The listing builds one solid part. Answer for the finished solid, in the listing's coordinates (mm). A direction names the side the tool comes from. Give positions to 0.01 mm unless a question says otherwise; leave off trailing zeros. Write each loop counter-clockwise with the first axis right and the second up, starting at its lowest first coordinate (ties: lowest second). Pieces come first, ordered by that corner, then holes. Notation, with made-up numbers: (-23, 19.25) - (10, 19.25) arc R34 ccw to (10, 50.25) - close; hole circle Ø4 at (81, 68.25). An arc over 180 degrees is marked (long way). Return JSON: item names as keys, results as strings.
Autodesk Inventor part; units mm, degrees
ref_plane "YZ Plane" through (0, 0, 0) normal (1, 0, 0) x (0, 1, 0)
ref_plane "XZ Plane" through (0, 0, 0) normal (0, 1, 0) x (-1, 0, 0)
ref_plane "XY Plane" through (0, 0, 0) normal (0, 0, 1) x (1, 0, 0)
sketch "スケッチ1" plane through (0, 0, 0) normal (0, 0, 1) x (1, 0, 0)
  circle A0 centre (0, 0) radius 17
  circle A1 centre (0, 0) radius 12
  circle A2 centre (0, -160) radius 12
  line L0 (-12, 0) -> (10.75, 0)
  line L1 (12, -160) -> (11, -160)
  circle A3 centre (0, -160) radius 17
  line L2 (-10, 24.6876) -> (10, 24.6876)
  line L3 (10, 24.6876) -> (10, -208.9864)
  line L4 (10, -208.9864) -> (-10, -208.9864)
  line L5 (-10, -208.9864) -> (-10, 24.6876)
  point P0 (-8, 8.9443)
  point P1 (12, 0)
  point P2 (0, -167.6676)
  point P3 (9.375, -145.8187)
  point P4 (-10.625, -146.7294)
  point P5 (-10.625, -13.2706)
  point P6 (9.375, -14.1813)
  point P7 (-0.625, 0)
  point P8 (-10, -13.7477)
  point P9 (-10, -146.2523)
  point P10 (10, -146.2523)
  point P11 (10, -13.7477)
  point P12 (10, -173.7477)
  point P13 (-10, -173.7477)
  point P14 (-10, 13.7477)
  point P15 (10, 13.7477)
  point P16 (-10, 6.6332)
  point P17 (-10, 0)
  point P18 (10, 0)
  point P19 (10, 6.6332)
  point P20 (-10, -6.6332)
  point P21 (10, -6.6332)
  point P22 (-10, -153.3668)
  point P23 (-10, -166.6332)
  point P24 (10, -166.6332)
  point P25 (10, -153.3668)
  dimension "d17" = 24
  dimension "d0" = 34
  dimension "d1" = 24
  dimension "d22" = 160
  dimension "d24" = 0
  dimension "d27" = 34
  dimension "d31" = 10
  dimension "d32" = 20
extrude "押し出し1" add sketch "スケッチ1" along normal blind 8 contours A0 L3 A1 | L3 A1 L5 A0 | L3 A3 L5 A0 | A0 L5 A1 L3 | L5 A1 A0 | L3 A2 L5 A3 | A3 L3 A2 | L5 A2 A3 | L5 A2 L3 A3
fillet "フィレット2" radius 5 4 edges at (-10, -146.2523, 4) (10, -146.2523, 4) (10, -13.7477, 4) (-10, -13.7477, 4)
equation "\"d17\" = d1"
equation "\"d31\" = 0.5 * d32"
equation "\"d23\" = 0.5 * d3"
properties part number "RP_Thigh-Link" material "アルミニウム7075"
Item 1: For faces 3 (the face through (10, -79, 4)), 4 (the face through (0.57, -176.99, 3.94)), 5 (the face through (-10.4, -14.13, 4.06)), determine the directions among +Z, -Z, +X, -X, +Y, -Y from which every point of the face is accessible in a straight line to the end or side of a thin tool.
Answer below:
{"face 3": "+Z, -Z, +X", "face 4": "+Z, -Z", "face 5": "+Z, -Z, -X"}
Item 2: The mould has two halves that part along Y. Classify faces 1 (the face through (0, -79, 0)), 2 (the face through (-10.426, -145.927, 4.056)): +Y half, -Y half, draft (parallel to the pull), parting line (faces both ways), or undercut.
Answer below:
{"face 1": "draft", "face 2": "undercut"}
Item 3: A cutting plane is placed at D-D on y = -102.5. Determine the outline of the cut face in (x, z), then the cut area to 3 significant figures.
Answer below:
{"outline": "(-10, 0) - (10, 0) - (10, 8) - (-10, 8) - close", "area": "160 mm²"}
Item 4: A cutting plane is placed at B-B on x = 0. Determine the outline of the cut face in (y, z).
Answer below:
{"outline": "(-177, 0) - (-172, 0) - (-172, 8) - (-177, 8) - close; (-148, 0) - (-12, 0) - (-12, 8) - (-148, 8) - close; (12, 0) - (17, 0) - (17, 8) - (12, 8) - close"}
Item 5: Consider L1, parallel to Y at x = 0, z = 4; L2, parallel to Y at x = 7.5, z = 7.5; L3, parallel to X at y = -160, z = 4. Determine where each line is inside the solid, lowest interval first.
Answer below:
{"L1": "y = -177 to -172, -148 to -12, 12 to 17", "L2": "y = -175.26 to -169.37, -150.63 to -9.37, 9.37 to 15.26", "L3": "x = -17 to -12, 12 to 17"}
Item 6: A cutting plane is placed at C-C on z = 6. Determine the outline of the cut face in (x, y), then the cut area to 3 significant figures.
Answer below:
{"outline": "(-11.59, -147.56) arc R17 ccw (long way) to (11.59, -147.56) arc R5 cw to (10, -143.91) - (10, -16.09) arc R5 cw to (11.59, -12.44) arc R17 ccw (long way) to (-11.59, -12.44) arc R5 cw to (-10, -16.09) - (-10, -143.91) arc R5 cw to start; hole circle Ø24 at (0, -160); hole circle Ø24 at (0, 0)", "area": "3,480 mm²"}
Item 7: Flat-ended cylindrical pins translate along their axes: P1, Ø3, axis at y = -99, z = 4.5, coming from the +X side; P2, Ø14.5, axis at x = 0, y = 0, coming from the +Z side (3 decimals); P3, Ø4, axis at x = 13.5, z = 5.5, coming from the -Y side; P4, Ø4, axis at y = -126.5, z = 5, coming from the -X side. Find the tip coordinate at first contact, or state that the pin passes through.
Answer below:
{"P1": "stops at x = 10", "P2": "passes through", "P3": "stops at y = -172.52", "P4": "stops at x = -10"}
Item 8: A cutting plane is placed at A-A on y = 0. Determine the outline of the cut face in (x, z).
Answer below:
{"outline": "(-17, 0) - (-12, 0) - (-12, 8) - (-17, 8) - close; (12, 0) - (17, 0) - (17, 8) - (12, 8) - close"}
